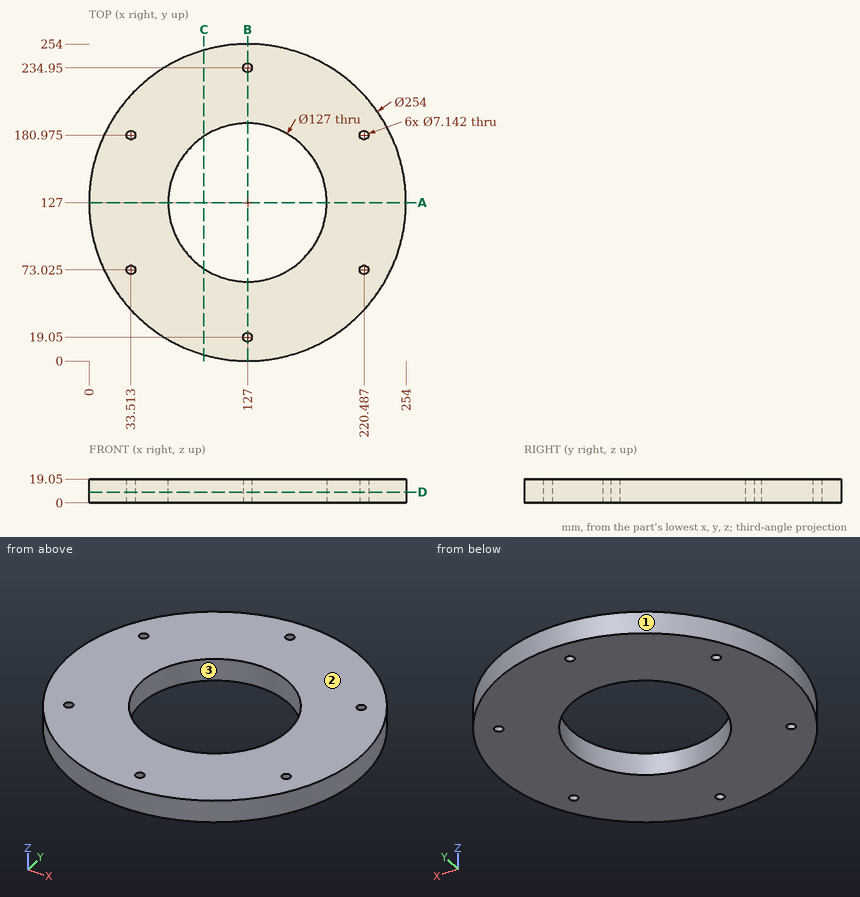
The figure shows three views and two pictorial views of one solid part (mm, origin at its lowest corner). Answer the questions. Round coordinates to 2 decimals unless told otherwise and drop trailing zeros. Order: outer loops, then holes, each group sorted by start corner. A loop starts at its lowest first (then second) coordinate and runs counter-clockwise, first axis right, second up. Notation, with made-up numbers: M -19.5,88.25 L 13.5,88.25 A21 ccw 13.5,121.25 Z; hole C -1.5,58 d3. An arc over 180 degrees is marked long. Answer in a Markdown table with one row per item. Add a question column.
1) Determine the mould class of the marked faces 1, 2 and 3 for opening direction Y: pulls with the +Y half, pulls with the -Y half, needs draft (parallel to the pull), parting line crosses it, or undercut.
2) The part is cut by section B-B on x = 127. Determine the outline of the cut face in (y, z).
3) The part is cut by section A-A on y = 127. Determine the outline of the cut face in (x, z).
4) The part is cut by section D-D on z = 8.5. Count the separate pieces of the cut face and the enclosed holes in it, plus the area to 3 significant figures.
5) Consider line 1 along Y through (x, z) = (127, 9.25); line 2 along X through (y, z) = (129, 4.75) (1 decimal); line 3 along Y through (x, z) = (156.5, 10) (1 decimal). Determine where each line is inside the solid, lowest interval first. Write a range as from..to.
6) Flat-ended cylindrical pins translate along their axes: pin 1 Ø4 at (x, z) = (154, 3) entering from +Y (1 decimal); pin 2 Ø5 at (y, z) = (222, 6.5) entering from +X; pin 3 Ø1 at (x, z) = (32.5, 8.5) entering from -Y. Find the tip coordinate at first contact, or state that the pin passes through.
7) The part is cut by section C-C on x = 92. Determine the outline of the cut face in (y, z).
Findings below:
| question | item | result |
|---|---|---|
| 1 | face 1 | parting line crosses it |
| 1 | face 2 | needs draft |
| 1 | face 3 | undercut |
| 2 | outline | M 0,0 L 15.48,0 L 15.48,19.05 L 0,19.05 Z; M 22.62,0 L 63.5,0 L 63.5,19.05 L 22.62,19.05 Z; M 190.5,0 L 231.38,0 L 231.38,19.05 L 190.5,19.05 Z; M 238.52,0 L 254,0 L 254,19.05 L 238.52,19.05 Z |
| 3 | outline | M 0,0 L 63.5,0 L 63.5,19.05 L 0,19.05 Z; M 190.5,0 L 254,0 L 254,19.05 L 190.5,19.05 Z |
| 4 | separate pieces | 1 |
| 4 | enclosed holes | 7 |
| 4 | area | 37,800 mm² |
| 5 | line 1 | y = 0..15.48, 22.62..63.5, 190.5..231.38, 238.52..254 |
| 5 | line 2 | x = 0..63.5, 190.5..254 |
| 5 | line 3 | y = 3.5..70.8, 183.2..250.5 |
| 6 | pin 1 | stops at y = 251.5 |
| 6 | pin 2 | stops at x = 214.02 |
| 6 | pin 3 | stops at y = 41.6 |
| 7 | outline | M 4.92,0 L 74.02,0 L 74.02,19.05 L 4.92,19.05 Z; M 179.98,0 L 249.08,0 L 249.08,19.05 L 179.98,19.05 Z |
